The model under review builds one solid part; all positions refer to its coordinate system, in mm. Face numbers are marked on the shaded views. A direction names the side the tool comes from. Coordinates: 2 decimals unless noted, no trailing zeros. Order: outer loops, then holes, each group sorted by start corner. A loop starts at its lowest first (then second) coordinate and runs counter-clockwise, first axis right, second up. Notation, with made-up numbers: (-10.75, 65) -> (34.25, 65) arc R24 ccw to (34.25, 94) -> close; hole circle Ø8 at (-4.75, 85). An arc over 180 degrees is marked (long way). Use one line per item in the form item = value. Start each with the question number.
(1) For the marked faces 4 and 5, list the 3-axis set-ups (+Z, -Z, +X, -X, +Y, -Y) from which the entire face can be reached by the end or side of a thin tool; tool diameter is ignored.
(2) Take a section at C-C (y = 3). State the section outline as (x, z) points (1 decimal).
(3) Mouldability with a two-part tool opening along X and no side actions: class the marked faces 1, 2 and 3 as +X half, -X half, draft (parallel to the pull), parting line (faces both ways), or undercut.
(4) Insertion check: pin 1 Ø2 at (y, z) = (19.5, -48.5) entering from +X; pin 2 Ø15 at (y, z) = (6, 11) entering from -X; pin 3 Ø4 at (y, z) = (1.5, 25) entering from +X. Each pin has a flat end and moves straight along its axis. Give the tip position at first contact, or say it passes through.
(5) Wall thickness on line 1 along Z through (x, y) = (-39, -12); line 2 along Z through (x, y) = (9, -11); line 3 along X through (y, z) = (-10, 6): over which ranges is each line inside the solid? List them lowest first.
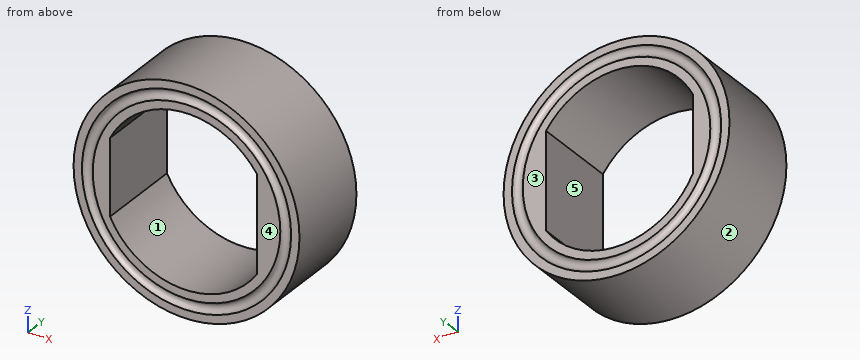
```python
from build123d import *

# Parameters (mm, degrees)
SKETCH1_R           = 65.0875
SKETCH1_R_2         = 49.2125
BOSS_EXTRUDE1_DEPTH = 25.4
SKETCH11_R          = 3.175
BOSS_EXTRUDE2_DEPTH = 50.8
BOSS_EXTRUDE4_DEPTH = 50.8


with BuildPart() as part:
    # Sketch1 → Boss-Extrude1 (new body, symmetric)
    with BuildSketch(Plane(origin=(0, 0, 0), x_dir=(1, 0, 0), z_dir=(0, 1, 0))):
        Circle(SKETCH1_R)
        Circle(SKETCH1_R_2, mode=Mode.SUBTRACT)
    extrude(amount=BOSS_EXTRUDE1_DEPTH, both=True)

    # Sketch11 → Cut-Revolve1 (revolve, cut)
    with BuildSketch(Plane.XY):
        with Locations((57.15, 26.035)):
            Circle(SKETCH11_R)
    cut_revolve1 = revolve(axis=Axis((0, 0, 0), (0, 1, 0)), mode=Mode.SUBTRACT)

    # Mirror1: Cut-Revolve1 across plane
    add(cut_revolve1.mirror(Plane.ZX), mode=Mode.SUBTRACT)

    # Sketch3 → Boss-Extrude2 (add, through all)
    with BuildSketch(Plane(origin=(0, 25.4, 0), x_dir=(1, 0, 0), z_dir=(0, 1, 0))):
        with BuildLine():
            Line((-44.0944, -21.853009973), (-44.0944, 21.853009973))
            ThreePointArc((-44.0944, 21.853009973), (-49.2125, 0), (-44.0944, -21.853009973))
        make_face()
    extrude(amount=-BOSS_EXTRUDE2_DEPTH)

    # Sketch6 → Boss-Extrude4 (add, through all)
    with BuildSketch(Plane(origin=(0, 25.4, 0), x_dir=(1, 0, 0), z_dir=(0, 1, 0))):
        with BuildLine():
            Line((40.64, 27.753568352), (40.64, -27.753568352))
            ThreePointArc((40.64, -27.753568352), (49.2125, 0), (40.64, 27.753568352))
        make_face()
    extrude(amount=-BOSS_EXTRUDE4_DEPTH)


solid = part.part
```
Findings:
q1.face_4 = +Z, -Z, +X, -X, -Y
q1.face_5 = +Y, -Y
q2.outline = circle Ø130.2 at (0, 0); hole (-44.1, -21.9) arc R49.2 ccw to (40.6, -27.8) -> (40.6, 27.8) arc R49.2 ccw to (-44.1, 21.9) -> close
q3.face_1 = undercut
q3.face_2 = parting line
q3.face_3 = draft
q4.pin_1 = 44.5
q4.pin_2 = -64.99
q4.pin_3 = 60.89
q5.line_1 = -52.11 to -30.01, 30.01 to 52.11
q5.line_2 = -64.46 to -48.38, 48.38 to 64.46
q5.line_3 = -64.81 to -44.09, 40.64 to 64.81
